Source: CAD feature listing. Evaluate the final solid. Frame: model axes, mm. Face numbers are marked on the shaded views. A direction names the side the tool comes from. Round coordinates to 2 decimals unless told otherwise and drop trailing zeros. Write each loop counter-clockwise with the first axis right and the second up, starting at its lowest first coordinate (ties: lowest second). Pieces come first, ordered by that corner, then holes. Notation, with made-up numbers: M 86.25,61.5 L 118.25,61.5 A23 ccw 118.25,77.5 Z; hole C -8,-11 d4. An arc over 180 degrees is marked long. Answer in a Markdown table with one row per item.
from build123d import *

# Parameters (mm, degrees)
SKETCH1_W      = 254
SKETCH1_H      = 127
EXTRUDE1_DEPTH = 25.4
FILLET1_R      = 12.7
FILLET2_R      = 1.27


with BuildPart() as part:
    # Sketch1 → Extrude1 (new body)
    with BuildSketch(Plane(origin=(0, 0, 0), x_dir=(1, 0, 0), z_dir=(0, 1, 0))):
        Rectangle(SKETCH1_W, SKETCH1_H)
    extrude(amount=EXTRUDE1_DEPTH)

    # Sketch3 → Revolve1 (revolve)
    with BuildSketch(Plane.XY, mode=Mode.PRIVATE) as revolve1_sk:
        Polygon((0, 127), (12.7, 127), (12.7, 101.6), (31.75, 101.6), (31.75, 76.2), (22.225, 76.2), (22.225, 25.4), (0, 25.4), align=None)
    revolve(revolve1_sk.sketch.rotate(Axis((0, 0, 0), (0, 1, 0)), 90), axis=Axis((0, 0, 0), (0, 1, 0)))

    # Fillet1
    fillet1_edges = [part.edges().sort_by_distance(p)[0] for p in [
        (-127, 12.7, -63.5),
        (127, 12.7, -63.5),
        (127, 12.7, 63.5),
        (-127, 12.7, 63.5),
    ]]
    fillet(fillet1_edges, radius=FILLET1_R)

    # Fillet2
    fillet2_edges = [part.edges().sort_by_distance(p)[0] for p in [
        (0, 25.4, 22.225),
        (0, 127, 12.7),
        (127, 25.4, 0),
        (0, 25.4, 63.5),
        (-127, 25.4, 0),
        (0, 25.4, -63.5),
        (-123.280256121, 25.4, 59.780256121),
        (-123.280256121, 25.4, -59.780256121),
        (123.280256121, 25.4, -59.780256121),
        (123.280256121, 25.4, 59.780256121),
    ]]
    fillet(fillet2_edges, radius=FILLET2_R)


solid = part.part
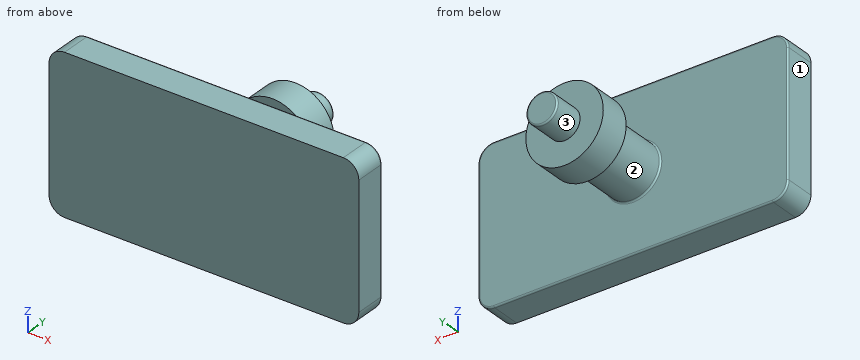
Q1. Access query for the marked faces 1, 2 and 3. Directions: +Z, -Z, +X, -X, +Y, -Y. A direction counts if a zero-diameter tool reaches every point of the face in a straight line with its end or side. Return the directions, or none.
Solutions:
| item | result |
|---|---|
| face 1 | +Z, -Z, -X, +Y, -Y |
| face 2 | none |
| face 3 | +Y |
Q2. Section A-A (x = 0). Return loops of the section in (y, z) (3 decimals).
Solutions:
| item | result |
|---|---|
| outline | M 0,-63.5 L 24.13,-63.5 A1.27 ccw 25.4,-62.23 L 25.4,-23.495 A1.27 cw 26.67,-22.225 L 76.2,-22.225 L 76.2,-31.75 L 101.6,-31.75 L 101.6,-12.7 L 125.73,-12.7 A1.27 ccw 127,-11.43 L 127,11.43 A1.27 ccw 125.73,12.7 L 101.6,12.7 L 101.6,31.75 L 76.2,31.75 L 76.2,22.225 L 26.67,22.225 A1.27 cw 25.4,23.495 L 25.4,62.23 A1.27 ccw 24.13,63.5 L 0,63.5 Z |
Q3. Contact query for flat-ended pins moving along their axis: pin 1 Ø1.5 at (y, z) = (76, 0) entering from +X; pin 2 Ø3 at (x, y) = (2.5, 39.5) entering from -Z; pin 3 Ø5 at (x, y) = (21.5, 93.5) entering from +Z. Output: stop coordinate, or through.
Solutions:
| item | result |
|---|---|
| pin 1 | stops at x = 31.75 |
| pin 2 | stops at z = -22.2 |
| pin 3 | stops at z = 25.44 |
Q4. Section B-B (z = 0). Return loops of the section in (x, y) (3 decimals), and give its area (3 significant figures).
Solutions:
| item | result |
|---|---|
| outline | M -127,0 L 127,0 L 127,24.13 A1.27 ccw 125.73,25.4 L 23.495,25.4 A1.27 cw 22.225,26.67 L 22.225,76.2 L 31.75,76.2 L 31.75,101.6 L 12.7,101.6 L 12.7,125.73 A1.27 ccw 11.43,127 L -11.43,127 A1.27 ccw -12.7,125.73 L -12.7,101.6 L -31.75,101.6 L -31.75,76.2 L -22.225,76.2 L -22.225,26.67 A1.27 cw -23.495,25.4 L -125.73,25.4 A1.27 ccw -127,24.13 Z |
| area | 11,000 mm2 |
Q5. Section D-D (x = 48.5). Return loops of the section in (y, z).
Solutions:
| item | result |
|---|---|
| outline | M 0,-63.5 L 24.13,-63.5 A1.27 ccw 25.4,-62.23 L 25.4,62.23 A1.27 ccw 24.13,63.5 L 0,63.5 Z |
Q6. Section C-C (y = 118.5). Return loops of the section in (x, z), and give its area (3 significant figures).
Solutions:
| item | result |
|---|---|
| outline | C 0,0 d25.4 |
| area | 507 mm2 |
Q7. Material intervals for probe 1 along Y at (x, z) = (-23.5, -58); probe 2 along Y at (x, z) = (14, 2.5); probe 3 along Z at (x, y) = (-20, 42), sorted ascending.
Solutions:
| item | result |
|---|---|
| probe 1 | y = 0 to 25.4 |
| probe 2 | y = 0 to 101.6 |
| probe 3 | z = -9.69 to 9.69 |
